from build123d import *

# Parameters (mm, degrees)
SKETCH1_R          = 2.6
BASE_FLANGE1_DEPTH = 3
FILLET_10_MM_R     = 10
FILLET_5_MM_R      = 5


# Sheet-metal steps are written as plain solids
with BuildPart() as part:
    # Sketch1 → Base-Flange1 (new body)
    with BuildSketch(Plane.XY):
        Polygon((-31, -0.559405941), (31, -0.559405941), (31, -25.559405941), (5, -55.559405941), (-5, -55.559405941), (-31, -25.559405941), align=None)
        with Locations((25, -7.559405941)):
            Circle(SKETCH1_R, mode=Mode.SUBTRACT)
        with Locations((-25, -7.559405941)):
            Circle(SKETCH1_R, mode=Mode.SUBTRACT)
        with BuildLine():
            Line((-2.6, -50.159405941), (-2.6, -44.959405941))
            ThreePointArc((-2.6, -44.959405941), (0, -42.359405941), (2.6, -44.959405941))
            Line((2.6, -44.959405941), (2.6, -50.159405941))
            ThreePointArc((2.6, -50.159405941), (0, -52.759405941), (-2.6, -50.159405941))
        make_face(mode=Mode.SUBTRACT)
        Polygon((0, -39.559405941), (19, -17.559405941), (19, -7.559405941), (-19, -7.559405941), (-19, -17.559405941), align=None, mode=Mode.SUBTRACT)
    extrude(amount=-BASE_FLANGE1_DEPTH)

    # fillet 10 mm
    fillet_10_mm_edges = [part.edges().sort_by_distance(p)[0] for p in [
        (31, -25.559405941, -1.5),
        (5, -55.559405941, -1.5),
        (-5, -55.559405941, -1.5),
        (-31, -25.559405941, -1.5),
        (-19, -17.559405941, -1.5),
        (19, -17.559405941, -1.5),
    ]]
    fillet(fillet_10_mm_edges, radius=FILLET_10_MM_R)

    # fillet 5 mm
    fillet_5_mm_edges = [part.edges().sort_by_distance(p)[0] for p in [
        (-31, -0.559405941, -1.5),
        (31, -0.559405941, -1.5),
        (0, -39.559405941, -1.5),
        (-19, -7.559405941, -1.5),
        (19, -7.559405941, -1.5),
    ]]
    fillet(fillet_5_mm_edges, radius=FILLET_5_MM_R)


solid = part.part
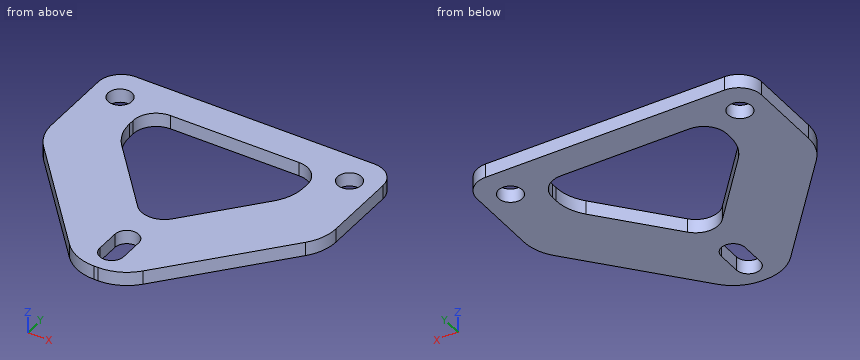
CAD build for the part. Positions are in the model's coordinates, mm. Give positions to 0.01 mm unless a question says otherwise; leave off trailing zeros. Loops run counter-clockwise (first coordinate to the right, second up) from the corner with the lowest first, then second, coordinate; pieces in that order, holes last. Notation, with made-up numbers: M -39.75,28 L -12.75,28 A15 cw -12.75,46 Z; hole C 75,-29.5 d10. An arc over 180 degrees is marked long. Answer in a Markdown table with one row per item. Add a question column.
Item 1: Band-saw the part on D-D on x = -21. Give the cut face in (y, z).
Item 2: Band-saw the part on B-B on z = -1.55. Give the cut face in (x, y), then the cut area to 3 significant figures.
Item 3: Band-saw the part on C-C on y = -26.5. Give the cut face in (x, z), then the cut area to 3 significant figures.
Item 4: Probe probe 1 along X at (y, z) = (-13, -2.45); probe 2 along Y at (x, z) = (2, -0.6); probe 3 along X at (y, z) = (-52, -0.7). List the from-to ranges inside material, lowest first.
Item 5: Band-saw the part on A-A on x = 6.5. Give the cut face in (y, z), then the cut area to 3 significant figures.
Item 6: Drop flat-ended pins along their axis: P1, Ø1, axis at x = 22.5, z = -2.5, coming from the -Y side; P2, Ø1.5, axis at x = 5, z = -0.5, coming from the -Y side; P3, Ø0.9, axis at y = -46.5, z = -1, coming from the -X side. Give the stop position or say it passes through.
Reply:
| question | item | result |
|---|---|---|
| 1 | outline | M -37.1,-3 L -0.56,-3 L -0.56,0 L -37.1,0 Z |
| 2 | outline | M -31,-21.83 A10 ccw -28.56,-28.38 L -7.99,-52.11 A10 ccw -0.43,-55.56 L 0.43,-55.56 A10 ccw 7.99,-52.11 L 28.56,-28.38 A10 ccw 31,-21.83 L 31,-5.56 A5 ccw 26,-0.56 L -26,-0.56 A5 ccw -31,-5.56 Z; hole C -25,-7.56 d5.2; hole M -19,-13.84 A10 ccw -16.57,-20.38 L -3.78,-35.18 A5 ccw 3.78,-35.18 L 16.57,-20.38 A10 ccw 19,-13.84 L 19,-12.56 A5 ccw 14,-7.56 L -14,-7.56 A5 ccw -19,-12.56 Z; hole M -2.6,-50.16 A2.6 ccw 2.6,-50.16 L 2.6,-44.96 A2.6 ccw -2.6,-44.96 Z; hole C 25,-7.56 d5.2 |
| 2 | area | 1,740 mm^2 |
| 3 | outline | M -29.84,-3 L -11.28,-3 L -11.28,0 L -29.84,0 Z; M 11.28,-3 L 29.84,-3 L 29.84,0 L 11.28,0 Z |
| 3 | area | 111 mm^2 |
| 4 | probe 1 | x = -31 to -19, 19 to 31 |
| 4 | probe 2 | y = -55.44 to -51.82, -43.3 to -36.49, -7.56 to -0.56 |
| 4 | probe 3 | x = -8.08 to -1.84, 1.84 to 8.08 |
| 5 | outline | M -53.51,-3 L -32.03,-3 L -32.03,0 L -53.51,0 Z; M -7.56,-3 L -0.56,-3 L -0.56,0 L -7.56,0 Z |
| 5 | area | 85.4 mm^2 |
| 6 | P1 | stops at y = -35.94 |
| 6 | P2 | stops at y = -54.8 |
| 6 | P3 | stops at x = -13.24 |
